Source: CAD feature listing. Evaluate the final solid. Frame: model axes, mm. Round coordinates to 2 decimals unless told otherwise and drop trailing zeros. Order: outer loops, then holes, each group sorted by start corner. A loop starts at its lowest first (then second) coordinate and runs counter-clockwise, first axis right, second up. Notation, with made-up numbers: (46, 44.25) -> (62, 44.25) arc R16 cw to (62, 74.25) -> close; hole circle Ø7 at (-6.5, 1.5). An arc over 180 degrees is marked (long way). Answer as CSV lines item,"result". Start each with the question number.
(1) Pull-direction query (Y, two-part tool) for faces 1 (the flat face through (22, 16, 0)), 2 (the cylindrical face through (39.45, 3.05, 0.99)), 3 (the flat face through (33.91, 27.42, 0.99)), 4 (the cylindrical face through (21.63, 46.95, 0.99)); classes: +Y half, -Y half, draft (parallel to the pull), parting line (faces both ways), or undercut.
(2) Contact query for a flat-ended pin moving along its axis: P1, Ø2.5, axis at x = 40.55, y = 3, coming from the -Z side. Output: stop coordinate, or through.
(3) Section query C-C (x = 26.5). Output: boundary loops of the cut face in (y, z), plus the area to 3 significant figures.
(4) Section query B-B (y = 8). Output: boundary loops of the cut face in (x, z), plus the area to 3 significant figures.
(5) Line query: line 1 along Y through (x, z) = (22, 1.2); line 2 along Y through (x, z) = (13.5, 0.4); line 3 along Y through (x, z) = (36, 1.75). Output: solid intervals per line, ascending. Write a range as from..to.
(6) Section query A-A (z = 1.45). Output: boundary loops of the cut face in (x, y).
```python
from build123d import *

# Parameters (mm, degrees)
ESQUISSE1_R        = 1.1
BOSS_EXTRU_1_DEPTH = 2


with BuildPart() as part:
    # Esquisse1 → Boss.-Extru.1 (new body)
    with BuildSketch(Plane.XY):
        Polygon((0, 0), (45, 0), (22.5, 55.621488653), align=None)
        with Locations((22.5, 3)):
            Circle(ESQUISSE1_R, mode=Mode.SUBTRACT)
        with Locations((14.031074433, 26.685744327)):
            Circle(ESQUISSE1_R, mode=Mode.SUBTRACT)
        with Locations((30.968925567, 26.685744327)):
            Circle(ESQUISSE1_R, mode=Mode.SUBTRACT)
        with Locations((4.449719092, 3)):
            Circle(ESQUISSE1_R, mode=Mode.SUBTRACT)
        with Locations((22.5, 47.621488653)):
            Circle(ESQUISSE1_R, mode=Mode.SUBTRACT)
        with Locations((40.550280908, 3)):
            Circle(ESQUISSE1_R, mode=Mode.SUBTRACT)
    extrude(amount=BOSS_EXTRU_1_DEPTH)


solid = part.part
```
Answer block:
1,face 1,"draft"
1,face 2,"undercut"
1,face 3,"+Y half"
1,face 4,"undercut"
2,P1,"z = 0"
3,outline,"(0, 0) -> (45.73, 0) -> (45.73, 2) -> (0, 2) -> close"
3,area,"91.5 mm2"
4,outline,"(3.24, 0) -> (41.76, 0) -> (41.76, 2) -> (3.24, 2) -> close"
4,area,"77.1 mm2"
5,line 1,"0..2.02, 3.98..46.64, 48.6..54.39"
5,line 2,"0..25.72, 27.65..33.37"
5,line 3,"0..22.25"
6,outline,"(0, 0) -> (45, 0) -> (22.5, 55.62) -> close; hole circle Ø2.2 at (4.45, 3); hole circle Ø2.2 at (14.03, 26.69); hole circle Ø2.2 at (22.5, 3); hole circle Ø2.2 at (22.5, 47.62); hole circle Ø2.2 at (30.97, 26.69); hole circle Ø2.2 at (40.55, 3)"
